Design review of the part built by this model. Coordinates are the model's own, in mm. Face numbers are marked on the shaded views. Give positions to 0.01 mm unless a question says otherwise; leave off trailing zeros. Write each loop counter-clockwise with the first axis right and the second up, starting at its lowest first coordinate (ties: lowest second). Pieces come first, ordered by that corner, then holes.
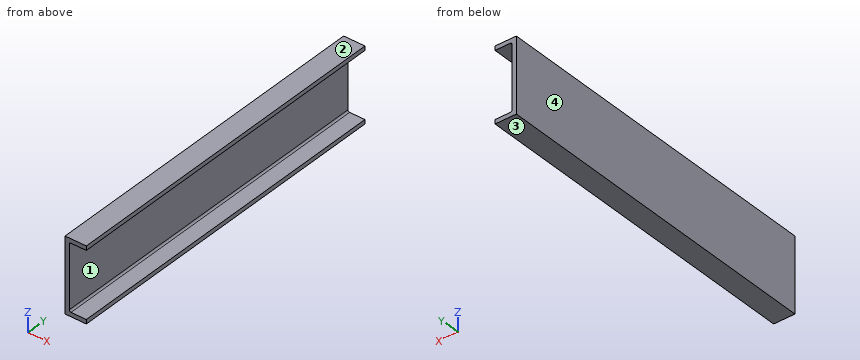
Autodesk Inventor part; units mm, degrees
ref_plane "YZ Plane" through (0, 0, 0) normal (1, 0, 0) x (0, 1, 0)
ref_plane "XZ Plane" through (0, 0, 0) normal (0, 1, 0) x (-1, 0, 0)
ref_plane "XY Plane" through (0, 0, 0) normal (0, 0, 1) x (1, 0, 0)
sketch "Sketch1" plane through (0, 0, 0) normal (1, 0, 0) x (0, 1, 0)
  line L0 (0, 0) -> (810, 0)
  line L1 (810, 0) -> (810, -175)
  line L2 (810, -175) -> (0, -175)
  line L3 (0, -175) -> (0, 0)
extrude "Extrusion1" add sketch "Sketch1" along normal blind 10
sketch "Sketch2" plane through (10, 0, 0) normal (1, 0, 0) x (0, 0, -1)
  line L0 (0, 810) -> (0, 0)
  line L1 (175, 0) -> (175, 810)
  line L2 (0, 0) -> (175, 0)
  line L3 (175, 0) -> (175, 10)
  line L4 (175, 10) -> (0, 10)
  line L5 (0, 10) -> (0, 0)
  line L6 (175, 810) -> (0, 810)
  line L7 (0, 10) -> (10, 10)
  line L8 (10, 10) -> (10, 810)
  line L9 (10, 810) -> (0, 810)
  line L10 (0, 810) -> (0, 10)
  line L11 (10, 810) -> (175, 810)
  line L12 (175, 810) -> (175, 800)
  line L13 (175, 800) -> (10, 800)
  line L14 (10, 800) -> (10, 810)
  line L15 (175, 800) -> (165, 800)
  line L16 (165, 800) -> (165, 10)
  line L17 (165, 10) -> (175, 10)
  line L18 (175, 10) -> (175, 800)
  dimension "d4" = 10
  dimension "d5" = 10
  dimension "d6" = 10
  dimension "d7" = 10
extrude "Extrusion2" add sketch "Sketch2" along normal blind 40
sketch "Sketch3" plane through (50, 0, 0) normal (1, 0, 0) x (0, 0, -1)
  line L0 (175, 0) -> (0, 0)
  line L1 (0, 810) -> (175, 810)
  line L2 (10, 0) -> (165, 0)
  line L3 (165, 0) -> (165, 810)
  line L4 (165, 810) -> (10, 810)
  line L5 (10, 810) -> (10, 0)
  dimension "d10" = 155
extrude "Extrusion3" cut sketch "Sketch3" against normal blind 40
fillet "Fillet1" radius 4 1 edges at (10, 405, -165)
fillet "Fillet2" radius 4 1 edges at (10, 405, -10)
equation "\"BendRadius\" = Thickness"
equation "\"BendReliefWidth\" = Thickness"
equation "\"BendReliefDepth\" = 0.5 * Thickness"
equation "\"CornerReliefSize\" = 4 * Thickness"
equation "\"MinimumRemnant\" = 2 * Thickness"
equation "\"TransitionRadius\" = BendRadius"
equation "\"JacobiRadiusSize\" = BendRadius"
equation "\"GapSize\" = Thickness"
properties part number "Base1"
(1) Consider section C-C, the plane z = -46. Give the boundary of the cut face in (x, y).
Resolved:
outline: (0, 0) - (10, 0) - (10, 810) - (0, 810) - close
(2) To check wall thickness, follow L1, parallel to Z at x = 15, y = 433.5; L2, parallel to X at y = 39.5, z = -112; L3, parallel to Z at x = 12, y = 111.5. State the ranges of each line that lie inside material, in increasing order.
Resolved:
L1: z = -175 to -165, -10 to 0
L2: x = 0 to 10
L3: z = -175 to -164.46, -10.54 to 0
(3) Consider section A-A, the plane x = 36. Give the boundary of the cut face in (y, z).
Resolved:
outline: (0, -175) - (810, -175) - (810, -165) - (0, -165) - close; (0, -10) - (810, -10) - (810, 0) - (0, 0) - close
(4) Clearance check with a flat-ended pin moving along its axis: P1, Ø6, axis at x = 15, z = -131, coming from the +Y side. State where the tip first meets the part, or that it passes through.
Resolved:
P1: passes through
(5) Mouldability with a two-part tool opening along Z and no side actions: class the marked faces 1, 2, 3 and 4 as pulls with the +Z half, pulls with the -Z half, needs draft (parallel to the pull), parting line crosses it, or undercut.
Resolved:
face 1: undercut
face 2: pulls with the +Z half
face 3: pulls with the -Z half
face 4: needs draft
(6) Consider section B-B, the plane y = 482.5. Give the boundary of the cut face in (x, z), then the cut area to 3 significant figures.
Resolved:
outline: (0, -175) - (50, -175) - (50, -165) - (14, -165) arc R4 cw to (10, -161) - (10, -14) arc R4 cw to (14, -10) - (50, -10) - (50, 0) - (0, 0) - close
area: 2,560 mm2
